Drawing for the job (mm, zero at the part's lowest x, y, z). A direction names the side the tool comes from. Give positions to 0.01 mm unless a question says otherwise; leave off trailing zeros. Order: outer loops, then holes, each group sorted by start corner. A loop starts at its lowest first (then second) coordinate and runs counter-clockwise, first axis right, second up. Notation, with made-up numbers: M 8,20 L 15,20 A5 cw 15,27 Z; hole C 44,8 d11. An arc over 180 degrees is marked long. Answer as a JSON object with one key per item and string values.
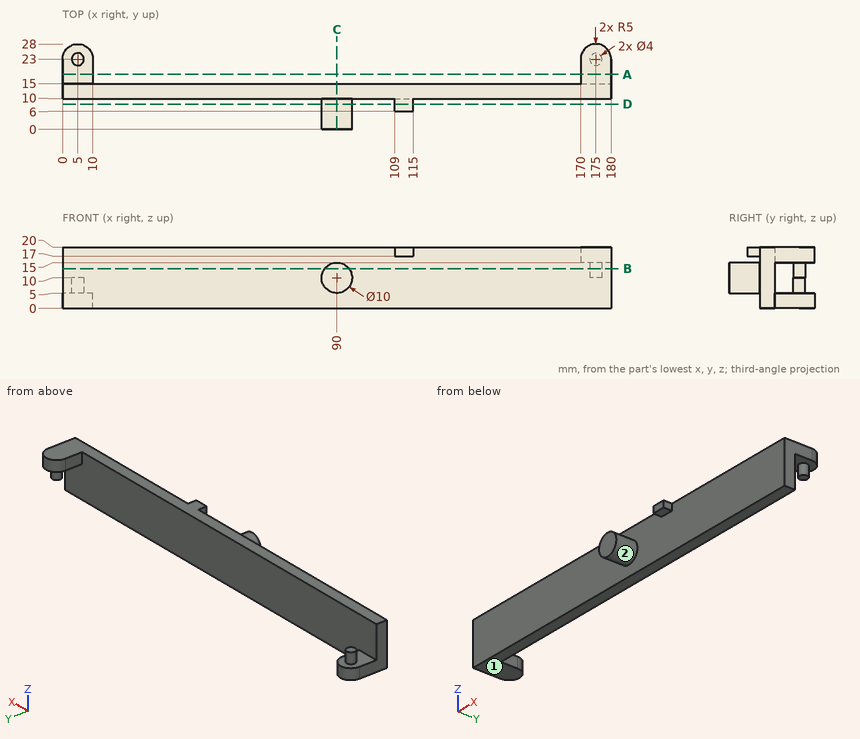
1. Cut at B-B on z = 13. Give the cut face in (x, y), plus the area to 3 significant figures.
Worked answers:
{"outline": "M 0,10 L 86,10 L 86,0 L 94,0 L 94,10 L 180,10 L 180,15 L 0,15 Z; C 175,23 d4", "area": "993 mm^2"}
2. Pin check, flat tips, straight feed: P1, Ø3, axis at x = 5.5, y = 23, coming from the +Z side; P2, Ø6, axis at x = 130, z = 4.5, coming from the +Y side; P3, Ø5, axis at x = 175.5, y = 24.5, coming from the -Z side. Stop position of each tip, or through.
Worked answers:
{"P1": "stops at z = 10", "P2": "stops at y = 15", "P3": "stops at z = 10"}
3. Cut at A-A on y = 18. Give the cut face in (x, z), plus the area to 3 significant figures.
Worked answers:
{"outline": "M 0,0 L 10,0 L 10,5 L 0,5 Z; M 170,15 L 180,15 L 180,20 L 170,20 Z", "area": "100 mm^2"}
4. Which spindle directions (+Z, -Z, +X, -X, +Y, -Y) get a long thin tool onto all of the face, cutting with end or side? Do the marked faces 1 and 2. Say none if no direction does.
Worked answers:
{"face 1": "-Z, +X, -X, +Y, -Y", "face 2": "-Y"}
5. Probe line 1 along Y through (x, z) = (113, 19); line 2 along Y through (x, z) = (48.5, 9.5); line 3 along Z through (x, y) = (90.5, 1.75). List the from-to ranges inside material, lowest first.
Worked answers:
{"line 1": "y = 6 to 15", "line 2": "y = 10 to 15", "line 3": "z = 5.03 to 14.97"}
6. Cut at D-D on y = 8.25. Give the cut face in (x, z), plus the area to 3 significant figures.
Worked answers:
{"outline": "C 90,10 d10; M 109,17 L 115,17 L 115,20 L 109,20 Z", "area": "96.5 mm^2"}
7. Cut at C-C on x = 90. Give the cut face in (y, z), plus the area to 3 significant figures.
Worked answers:
{"outline": "M 0,5 L 10,5 L 10,0 L 15,0 L 15,20 L 10,20 L 10,15 L 0,15 Z", "area": "200 mm^2"}
